Read the model definition and answer for the solid it produces. Units are mm, in the model's axes. A direction names the side the tool comes from. Coordinates: 2 decimals unless noted, no trailing zeros. Loops run counter-clockwise (first coordinate to the right, second up) from the corner with the lowest first, then second, coordinate; pieces in that order, holes last. Notation, with made-up numbers: (-40, 5.25) - (18, 5.25) arc R18 ccw to (18, 26.25) - close; hole circle Ø4 at (-24, -22.5). An arc over 180 degrees is marked (long way). One line per question, with ' | ' between items. Start each with the question number.
```python
from build123d import *
from OCP.BRepFilletAPI import BRepFilletAPI_MakeChamfer

# Parameters (mm, degrees)
BODY_DEPTH                 = 15
SHAPE_CUT_DEPTH            = 67.708320321
RAIL_CUTOUT_DEPTH          = 67.708320321
GUIDING_SCREWS_START       = 3.087719198
GUIDING_SCREWS_OUTLINE_R   = 4
GUIDING_SCREWS_DEPTH       = 11.912280802
GUIDING_SCREWS_START_2     = 15
GUIDING_SCREWS_2_OUTLINE_R = 2.15
GUIDING_SCREWS_2_DEPTH     = 10
SKETCH6_R                  = 1.4
TONG_TIP_CHAMFERS_SIZE     = 2
TONG_TIP_CHAMFERS_SIZE2    = 2.200726077


# Read off the part's stored shape, not the designer's step: guiding_screws
with BuildPart() as part:
    # Sketch1 → body (new body)
    with BuildSketch(Plane.XY):
        Polygon((0, 0), (25, 0), (25, -30), (22, -33), (22, -60), (8, -60), (3, -3), align=None)
    extrude(amount=BODY_DEPTH)

    # Sketch2 → shape_cut (cut, through all)
    with BuildSketch(Plane(origin=(25, 0, 0), x_dir=(0, 0, -1), z_dir=(1, 0, 0))):
        Polygon((-15, 0), (-12.5, -2.5), (-12.5, -30), (-11.5, -33), (-11.5, -60), (-15, -60), align=None)
        Polygon((0, 0), (-2.5, -2.5), (-2.5, -30), (-3.5, -33), (-3.5, -60), (0, -60), align=None)
    extrude(amount=-SHAPE_CUT_DEPTH, mode=Mode.SUBTRACT)

    # Sketch3 → rail_cutout (cut, through all)
    with BuildSketch(Plane(origin=(25, 0, 0), x_dir=(0, 0, -1), z_dir=(1, 0, 0))):
        Polygon((-10, 0), (-5, 0), (-6, -2), (-9, -2), align=None)
    extrude(amount=-RAIL_CUTOUT_DEPTH, mode=Mode.SUBTRACT)

    # guiding_screws outline → guiding_screws (cut)
    with BuildSketch(Plane.YZ.offset(GUIDING_SCREWS_START)):
        with Locations((-24, 7.5)):
            Circle(GUIDING_SCREWS_OUTLINE_R)
        with Locations((-8, 7.5)):
            Circle(GUIDING_SCREWS_OUTLINE_R)
    extrude(amount=GUIDING_SCREWS_DEPTH, mode=Mode.SUBTRACT)

    # guiding_screws 2 outline → guiding_screws 2 (cut)
    with BuildSketch(Plane.YZ.offset(GUIDING_SCREWS_START_2)):
        with Locations((-24, 7.5)):
            Circle(GUIDING_SCREWS_2_OUTLINE_R)
        with Locations((-8, 7.5)):
            Circle(GUIDING_SCREWS_2_OUTLINE_R)
    extrude(amount=GUIDING_SCREWS_2_DEPTH, mode=Mode.SUBTRACT)

    # Sketch6 → rope_connector_cutout (revolve, cut)
    with BuildSketch(Plane(origin=(25, 0, 0), x_dir=(0, 0, -1), z_dir=(1, 0, 0)), mode=Mode.PRIVATE) as rope_connector_cutout_sk:
        with Locations((-7.5, -12.2)):
            Circle(SKETCH6_R)
    revolve(rope_connector_cutout_sk.sketch.rotate(Axis((25, -16, 12.5), (0, 0, -1)), 270), axis=Axis((25, -16, 12.5), (0, 0, -1)), mode=Mode.SUBTRACT)

    # tong_tip_chamfers: one chamfer whose edges measure the first distance from different faces: ONE call of the kernel's chamfer builder (chamfer() names one face for all edges)
    tong_tip_chamfers_edges_1 = [part.edges().sort_by_distance(p)[0] for p in [
        (22, -60, 7.5),
    ]]
    tong_tip_chamfers_edges_2 = [part.edges().sort_by_distance(p)[0] for p in [
        (8, -60, 7.5),
    ]]
    tong_tip_chamfers_side_2 = [part.faces().sort_by_distance(p)[0] for p in [
        (5.65880617, -33.310390339, 7.5),
    ]]
    tong_tip_chamfers = BRepFilletAPI_MakeChamfer(part.part.solid().wrapped)
    for e in tong_tip_chamfers_edges_1:
        tong_tip_chamfers.Add(TONG_TIP_CHAMFERS_SIZE, e.wrapped)
    for e in tong_tip_chamfers_edges_2:
        tong_tip_chamfers.Add(TONG_TIP_CHAMFERS_SIZE, TONG_TIP_CHAMFERS_SIZE2, e.wrapped, tong_tip_chamfers_side_2[0].wrapped)  # the first distance lies on this face
    add(Compound.cast(tong_tip_chamfers.Shape()), mode=Mode.REPLACE)

    # Sketch9 → tong_tip_hole (revolve, cut)
    with BuildSketch(Plane(origin=(16, -52, 11.5), x_dir=(0, -1, 0), z_dir=(1, 0, 0))):
        Polygon((0, 0), (0, 8), (2, 8), (1.7, 7.7), (1.7, 0.3), (2, 0), align=None)
    revolve(axis=Axis((16, -52, 17.85), (0, 0, -1)), mode=Mode.SUBTRACT)


solid = part.part
```
1) Given pin 1 Ø2 at (x, y) = (5.5, -32.5) entering from -Z; pin 2 Ø2 at (x, y) = (8.5, -30) entering from +Z; pin 3 Ø4 at (y, z) = (-24, 6) entering from -X, each flat-ended and moving along its own axis, determine where each tip first touches the part or whether it passes through.
2) The part is cut by section B-B on z = 7.5. Count the separate pieces of the cut face and the enclosed holes in it, and give its area (3 significant figures).
3) The part is cut by section A-A on x = 16. Write down the section's boundary in (y, z), and give its area (3 significant figures).
4) Find the intervals of material crossed by line 1 along Z through (x, y) = (20.5, -24); line 2 along Z through (x, y) = (8.25, -8); line 3 along Y through (x, z) = (11.25, 4), in increasing order. Write a range as from..to.
5) The part is cut by section C-C on y = -52. Write down the section's boundary in (x, z).
6) Which of the six approach directions +Z, -Z, +X, -X, +Y, -Y give full straight-line access (tool end or side, diameter ignored) to faces 1 (the flat face through (12.7, -1, 9.5)), 2 (the flat face through (14, -46, 3.5)), 3 (the flat face through (15, -22, 6))?
7) The mould has two halves that part along Y. Classify faces 4 (the flat face through (25, -15, 9)), 5 (the flat face through (2.2, -2.2, 7.4)), 6 (the cylindrical face through (15.93, -50.3, 7.55)): released by +Y, released by -Y, zero draft, split by the parting line, or undercut.
8) The part is cut by section D-D on y = -8. Write down the section's boundary in (x, z).
Answer below:
1) pin 1: z = 3 | pin 2: z = 12.5 | pin 3: x = 15
2) separate pieces: 4 | enclosed holes: 1 | area: 742 mm2
3) outline: (-60, 3.5) - (-54, 3.5) - (-53.7, 3.8) - (-53.7, 11.2) - (-54, 11.5) - (-60, 11.5) - close; (-50.3, 3.8) - (-50, 3.5) - (-33, 3.5) - (-30, 2.5) - (-2.5, 2.5) - (0, 0) - (0, 5) - (-2, 6) - (-2, 9) - (0, 10) - (0, 15) - (-2.5, 12.5) - (-30, 12.5) - (-33, 11.5) - (-50, 11.5) - (-50.3, 11.2) - close; hole circle Ø4.3 at (-24, 7.5); hole circle Ø4.3 at (-8, 7.5) | area: 485 mm2
4) line 1: 2.5..5.35, 9.65..12.5 | line 2: 2.5..3.5, 11.5..12.5 | line 3: -60..-25.94, -22.06..-9.94, -6.06..0
5) outline: (7.3, 3.5) - (14, 3.5) - (14.3, 3.8) - (14.3, 11.2) - (14, 11.5) - (7.3, 11.5) - close; (17.7, 3.8) - (18, 3.5) - (22, 3.5) - (22, 11.5) - (18, 11.5) - (17.7, 11.2) - close
6) face 1: +X, -X, +Y | face 2: -Z, +X, -X, -Y | face 3: -X
7) face 4: zero draft | face 5: released by -Y | face 6: undercut
8) outline: (3.44, 2.5) - (25, 2.5) - (25, 5.35) - (15, 5.35) - (15, 3.5) - (3.44, 3.5) - close; (3.44, 11.5) - (15, 11.5) - (15, 9.65) - (25, 9.65) - (25, 12.5) - (3.44, 12.5) - close
